from build123d import *

# Parameters (mm, degrees)
F0_W     = 200
F0_H     = 300
F1_DEPTH = 5
F2_R     = 1.5875
F3_DEPTH = 5.001
F4_R     = 1.5875
F5_DEPTH = 25
F7_DEPTH = 5
F8_R     = 2.5
F9_DEPTH = 25


with BuildPart() as f1:
    # F0 (on Top) → F1 (new body)
    with BuildSketch(Plane.XY):
        Rectangle(F0_W, F0_H)
    extrude(amount=F1_DEPTH)

    # F2 (on face) → F3 (cut, through all)
    with BuildSketch(Plane.XY.offset(5)):
        Circle(F2_R)
        with Locations((0, -35.650707)):
            Circle(F2_R)
        with Locations((-60.544926, 6.347642)):
            Circle(F2_R)
        with Locations((-35, 61.605559)):
            Circle(F2_R)
        with Locations((0, 136.605559)):
            Circle(F2_R)
    extrude(amount=-F3_DEPTH, mode=Mode.SUBTRACT)

    # F4 (on face) → F5 (cut)
    with BuildSketch(Plane.XY.offset(5)):
        Polygon((-70, -50), (-70, 150), (-100, 150), (-100, -150), (100, -150), (100, 150), (10, 150), (10, -50), align=None)
        Circle(F4_R)
        with Locations((0, -35.650707)):
            Circle(F4_R)
        with Locations((-60.544926, 6.347642)):
            Circle(F4_R)
        with Locations((-35, 61.605559)):
            Circle(F4_R)
        with Locations((0, 136.605559)):
            Circle(F4_R)
    extrude(amount=-F5_DEPTH, mode=Mode.SUBTRACT)

    # F6 (on face) → F7 (join)
    with BuildSketch(Plane.XY.offset(5)):
        with BuildLine():
            ThreePointArc((-33.4125, 61.605559), (-33.877468, 60.483027), (-35, 60.018059))
            Line((-35, 60.018059), (-35, 46.803687))
            Line((-35, 46.803687), (0, 84.999484))
            Line((0, 84.999484), (0, 99.801357))
            Line((0, 99.801357), (-33.927501, 62.775987))
            ThreePointArc((-33.927501, 62.775987), (-33.546943, 62.244919), (-33.4125, 61.605559))
        make_face()
        with BuildLine():
            Line((-35, 46.803687), (-35, 60.018059))
            ThreePointArc((-35, 60.018059), (-35.341033, 60.055123), (-35.666142, 60.164583))
            Line((-35.666142, 60.164583), (-48.809552, 31.733206))
            Line((-48.809552, 31.733206), (-35, 46.803687))
        make_face()
        with BuildLine():
            ThreePointArc((-36.072499, 60.435131), (-36.170428, 62.678058), (-33.927501, 62.775987))
            Line((-33.927501, 62.775987), (0, 99.801357))
            Line((0, 99.801357), (0, 109.801357))
            ThreePointArc((0, 109.801357), (-4.027467, 108.954471), (-7.372773, 106.557259))
            Line((-7.372773, 106.557259), (-108.711305, -4.034342))
            ThreePointArc((-108.711305, -4.034342), (-108.094433, -18.163017), (-93.965758, -17.546146))
            Line((-93.965758, -17.546146), (-48.809552, 31.733206))
            Line((-48.809552, 31.733206), (-35.666142, 60.164583))
            ThreePointArc((-35.666142, 60.164583), (-35.879783, 60.284144), (-36.072499, 60.435131))
        make_face()
        with BuildLine():
            Line((0, 109.801357), (0, 99.801357))
            Line((0, 99.801357), (0, 84.999484))
            Line((0, 84.999484), (7.372773, 93.045455))
            ThreePointArc((7.372773, 93.045455), (9.153115, 103.828823), (0, 109.801357))
        make_face()
    extrude(amount=-F7_DEPTH)

    # F8 (on face) → F9 (cut)
    with BuildSketch(Plane.XY.offset(5)):
        with Locations((-101.016482, -10.755953)):
            Circle(F8_R)
    extrude(amount=-F9_DEPTH, mode=Mode.SUBTRACT)


solid = f1.part
The listing builds one solid part. Answer for the finished solid, in the listing's coordinates (mm). A direction names the side the tool comes from. Round coordinates to 2 decimals unless told otherwise and drop trailing zeros. Order: outer loops, then holes, each group sorted by start corner. A loop starts at its lowest first (then second) coordinate and runs counter-clockwise, first axis right, second up. Notation, with made-up numbers: (-19, 12) - (13, 12) arc R32 ccw to (13, 48) - close; hole circle Ø10 at (-31, 32.5). An arc over 180 degrees is marked (long way). Write item = value, one per line. Start each with the question number.
1) Straight lines are drawn through the part: L1, parallel to Y at x = 0, z = 1.6; L2, parallel to Y at x = -1, z = 2.1; L3, parallel to X at y = 80.5, z = 1. For each, find the intervals that lie inside material, in ascending order.
2) Given pin 1 (2 mm diameter, centred on y = -17, z = 3.5, fed in from -X); pin 2 (2.5 mm diameter, centred on y = -30, z = 1.5, fed in from -X), each flat-ended and moving along its own axis, determine where each tip first touches the part or whether it passes through.
3) Section B-B, the plane y = -31.5 is taken. Write down the section's boundary in (x, z), plus the area to 3 significant figures.
4) Section C-C, the plane x = -82.5 is taken. Write down the section's boundary in (y, z), plus the area to 3 significant figures.
5) Section A-A, the plane z = 1.65 is taken. Write down the section's boundary in (x, y) (1 decimal).
6) For a pull along X with two mould halves and no side action, classify faces 1 (the flat face through (-70, -21, 3)), 2 (the flat face through (-38, 51, 0)), 3 (the flat face through (-89.085, 17.384, 2.535)) as released by +X, released by -X, zero draft, split by the parting line, or undercut.
7) For faces 4 (the flat face through (-70, 93, 3)), 5 (the flat face through (-82.15, -4.65, 2.54)), 6 (the flat face through (-38, 51, 5)), determine the directions among +Z, -Z, +X, -X, +Y, -Y from which every point of the face is accessible in a straight line to the end or side of a thin tool.
Results list:
q1.L1 = -50 to -37.24, -34.06 to -1.59, 1.59 to 135.02, 138.19 to 150
q1.L2 = -50 to -36.88, -34.42 to -1.23, 1.23 to 135.37, 137.84 to 150
q1.L3 = -70 to 10
q2.pin_1 = -109.87
q2.pin_2 = -70
q3.outline = (-70, 0) - (10, 0) - (10, 5) - (-70, 5) - close
q3.area = 400 mm^2
q4.outline = (-5.03, 0) - (24.57, 0) - (24.57, 5) - (-5.03, 5) - close
q4.area = 148 mm^2
q5.outline = (-108.7, -4) arc R10 ccw to (-94, -17.5) - (-70, 8.6) - (-70, -50) - (10, -50) - (10, 150) - (-70, 150) - (-70, 38.2) - close; hole circle Ø5 at (-101, -10.8); hole circle Ø3.2 at (-60.5, 6.3); hole (-36.1, 60.4) arc R1.6 ccw to (-35.7, 60.2) arc R1.6 ccw to (-35, 60) arc R1.6 ccw (long way) to start; hole circle Ø3.2 at (0, -35.7); hole circle Ø3.2 at (0, 0); hole circle Ø3.2 at (0, 136.6)
q6.face_1 = undercut
q6.face_2 = zero draft
q6.face_3 = released by -X
q7.face_4 = +Z, -Z, -X, +Y
q7.face_5 = +Z, -Z, -Y
q7.face_6 = +Z, +X, -X, +Y, -Y
